from build123d import *

# Parameters (mm, degrees)
F0_W     = 100
F0_H     = 50
F1_DEPTH = 6
F2_R     = 3
F3_DEPTH = 10
F4_R     = 2
F5_R     = 3
F6_DEPTH = 5


with BuildPart() as f1:
    # F0 (on Front) → F1 (new body)
    with BuildSketch(Plane.XZ):
        Rectangle(F0_W, F0_H)
    extrude(amount=F1_DEPTH)

    # F2 (on face) → F3 (join)
    with BuildSketch(Plane.XZ.offset(6)):
        with Locations((-19.068, 0)):
            Circle(F2_R)
        with Locations((19.068, 0)):
            Circle(F2_R)
    extrude(amount=F3_DEPTH)

    # F4
    f4_edges = [f1.edges().sort_by_distance(p)[0] for p in [
        (50, -6, 0),
        (0, -6, -25),
        (0, -6, 25),
        (-50, -6, 0),
        (-22.068, -6, 0),
        (16.068, -6, 0),
    ]]
    fillet(f4_edges, radius=F4_R)

    # F5 (on face) → F6 (join)
    with BuildSketch(Plane.XZ.offset(16)):
        with Locations((-19.068, 0)):
            Circle(F5_R)
    extrude(amount=F6_DEPTH)


solid = f1.part
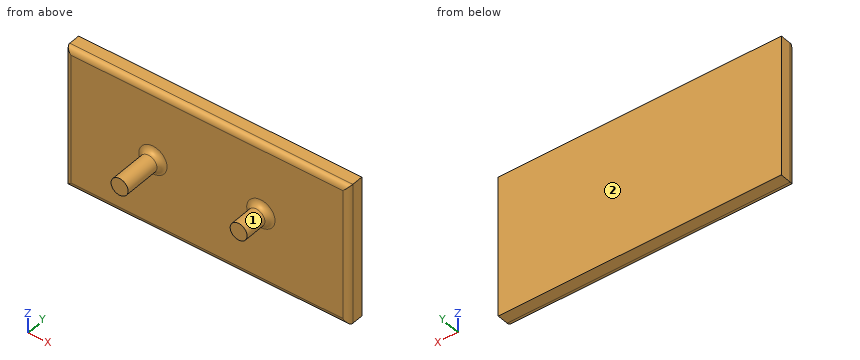
Work out the finished part from the listing and answer in its coordinate system (mm). Face numbers are marked on the shaded views. Round coordinates to 2 decimals unless told otherwise and drop trailing zeros. Order: outer loops, then holes, each group sorted by start corner. A loop starts at its lowest first (then second) coordinate and runs counter-clockwise, first axis right, second up. Notation, with made-up numbers: M -18.75,-36 L 40.25,-36 A19 cw 40.25,-20 Z; hole C -19.5,9.25 d3. An arc over 180 degrees is marked long. Put each result on its own line as item: value. Start each with the question number.
Q1. Section A-A, the plane z = 21.5 is taken. Write down the section's boundary in (x, y).
Q2. Section C-C, the plane x = 28 is taken. Write down the section's boundary in (y, z), and give its area (3 significant figures).
Q3. Flat-ended cylindrical pins translate along their axes: pin 1 (10 mm diameter, centred on y = -15, z = 4.5, fed in from -X); pin 2 (5 mm diameter, centred on y = -7, z = -12.5, fed in from -X); pin 3 (12 mm diameter, centred on y = -8.5, z = -10, fed in from -X); pin 4 (6 mm diameter, centred on x = -26, y = -11.5, fed in from +Z). Find the tip coordinate at first contact, or state that the pin passes through.
Q4. Section D-D, the plane z = 0 is taken. Write down the section's boundary in (x, y).
Q5. Straight lines are drawn through the part: L1, parallel to Y at x = 10, z = -17; L2, parallel to X at y = -5, z = -13; L3, parallel to Z at x = -17, y = -20. For each, find the intervals that lie inside material, in ascending order. Write a range as [from, to].
Q6. Section B-B, the plane y = -14.5 is taken. Write down the section's boundary in (x, z).
Q7. For a pull along X with two mould halves and no side action, classify the marked faces 1 and 2 as pulls with the +X half, pulls with the -X half, needs draft (parallel to the pull), parting line crosses it, or undercut.
Findings below:
1. outline: M -50,-4 A2 ccw -48,-6 L 48,-6 A2 ccw 50,-4 L 50,0 L -50,0 Z
2. outline: M -6,-23 A2 ccw -4,-25 L 0,-25 L 0,25 L -4,25 A2 ccw -6,23 Z
2. area: 298 mm^2
3. pin 1: stops at x = -22.07
3. pin 2: stops at x = -49.94
3. pin 3: stops at x = -50
3. pin 4: passes through
4. outline: M -50,-4 A2 ccw -48,-6 L -24.07,-6 A2 cw -22.07,-8 L -22.07,-21 L -16.07,-21 L -16.07,-8 A2 cw -14.07,-6 L 14.07,-6 A2 cw 16.07,-8 L 16.07,-16 L 22.07,-16 L 22.07,-8 A2 cw 24.07,-6 L 48,-6 A2 ccw 50,-4 L 50,0 L -50,0 Z
5. L1: y = [-6, 0]
5. L2: x = [-49.73, 49.73]
5. L3: z = [-2.17, 2.17]
6. outline: C -19.07,0 d6; C 19.07,0 d6
7. face 1: undercut
7. face 2: needs draft
